from build123d import *

# Parameters (mm, degrees)
BOSS_EXTRUDE1_DEPTH = 15
SHELL2_T            = 6
CUT_EXTRUDE1_REACH  = 17
SKETCH2_R           = 15
CUT_EXTRUDE2_REACH  = 42
SKETCH3_R           = 2.25
SKETCH5_R           = 5.54
CUT_EXTRUDE3_DEPTH  = 21


with BuildPart() as part:
    # Sketch1 → Boss-Extrude1 (new body)
    with BuildSketch(Plane.XY):
        with BuildLine():
            Line((-25, 0), (-25, -15))
            Line((-25, -15), (25, -15))
            Line((25, -15), (25, 0))
            ThreePointArc((25, 0), (0, 25), (-25, 0))
        make_face()
    extrude(amount=BOSS_EXTRUDE1_DEPTH)

    # Shell2 (no face opened: a closed hollow body)
    add(offset(amount=-SHELL2_T, mode=Mode.PRIVATE), mode=Mode.SUBTRACT)

    # Sketch2 → Cut-Extrude1 (cut, up to next)
    with BuildSketch(Plane.XY.offset(15), mode=Mode.PRIVATE) as cut_extrude1_sk1:
        with Locations((0, -5)):
            Circle(SKETCH2_R)
    cut_extrude1_tool1 = extrude(cut_extrude1_sk1.sketch, amount=-CUT_EXTRUDE1_REACH, mode=Mode.PRIVATE) & part.part
    add(cut_extrude1_tool1.solids().sort_by_distance((0, -5, 15))[0], mode=Mode.SUBTRACT)

    # Sketch3 → Cut-Extrude2 (cut, up to next)
    with BuildSketch(Plane(origin=(0, 25, 0), x_dir=(1, 0, 0), z_dir=(0, 1, 0)), mode=Mode.PRIVATE) as cut_extrude2_sk1:
        with Locations((-19, -7.5)):
            Circle(SKETCH3_R)
    cut_extrude2_tool1 = extrude(cut_extrude2_sk1.sketch, amount=-CUT_EXTRUDE2_REACH, mode=Mode.PRIVATE) & part.part
    add(cut_extrude2_tool1.solids().sort_by_distance((-19, 25, 7.5))[0], mode=Mode.SUBTRACT)
    # Sketch3 → Cut-Extrude2 (cut, up to next)
    with BuildSketch(Plane(origin=(0, 25, 0), x_dir=(1, 0, 0), z_dir=(0, 1, 0)), mode=Mode.PRIVATE) as cut_extrude2_sk2:
        with Locations((19, -7.5)):
            Circle(SKETCH3_R)
    cut_extrude2_tool2 = extrude(cut_extrude2_sk2.sketch, amount=-CUT_EXTRUDE2_REACH, mode=Mode.PRIVATE) & part.part
    add(cut_extrude2_tool2.solids().sort_by_distance((19, 25, 7.5))[0], mode=Mode.SUBTRACT)

    # Sketch5 → Cut-Extrude3 (cut)
    with BuildSketch(Plane(origin=(0, 25, 0), x_dir=(1, 0, 0), z_dir=(0, 1, 0))):
        with Locations((19, -7.5)):
            Circle(SKETCH5_R)
        with Locations((-19, -7.5)):
            Circle(SKETCH5_R)
    extrude(amount=-CUT_EXTRUDE3_DEPTH, mode=Mode.SUBTRACT)


solid = part.part
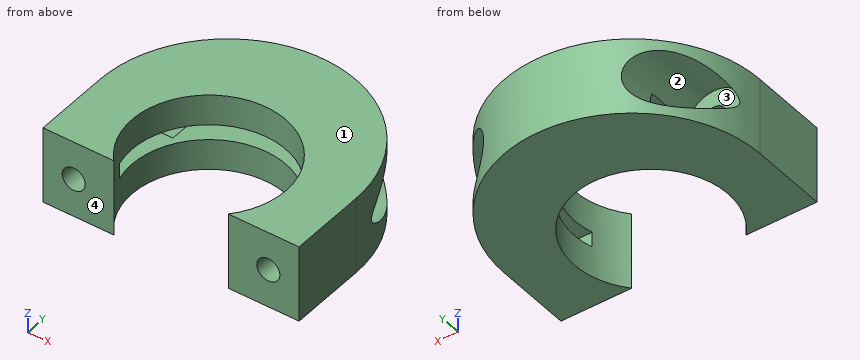
Here's how the part is built. I have some questions about the finished solid (model axes, mm). Face numbers are marked on the shaded views. Round coordinates to 2 decimals unless told otherwise and drop trailing zeros. Loops run counter-clockwise (first coordinate to the right, second up) from the corner with the lowest first, then second, coordinate; pieces in that order, holes last. Notation, with made-up numbers: M 41,-23 L 88,-23 A22 cw 88,1 Z; hole C 46,86.25 d6. An arc over 180 degrees is marked long. Write each question's results on one line, items separated by ' | '. Start each with the question number.
(1) I want a section at C-C (z = 7.5). Please give me the cut outline in (x, y), then the cut area to 3 significant figures.
(2) I want a section at D-D (x = -19). Please give me the cut outline in (y, z).
(3) I want a section at B-B (x = 0). Please give me the cut outline in (y, z).
(4) Thinking about a two-plate mould opening in Z: for the marked faces 1, 2, 3 and 4, which applies, pulls with the +Z half, pulls with the -Z half, needs draft (parallel to the pull), parting line crosses it, or undercut?
(5) I want a section at A-A (y = -5). Please give me the cut outline in (x, z), then the cut area to 3 significant figures.
(6) If I drill on probe 1 along X at (y, z) = (-5.5, 7.5); probe 2 along X at (y, z) = (3.5, 5.5); probe 3 along Z at (x, y) = (-19, -6.5), over which ranges is the centre line in solid material (lowest first)? Write a range as from..to.
(7) Will these pins go through, and if not, where does the flat tip stop? P1, Ø0.9, axis at x = -15.5, z = 8, coming from the +Y side; P2, Ø1, axis at y = 21, z = 5, coming from the +X side; P3, Ø5.5, axis at x = 18, z = 5.5, coming from the +Y side; P4, Ø24, axis at x = 0, y = -5, coming from the -Z side.
Solved:
1) outline: M -25,-15 L -21.25,-15 L -21.25,4 L -24.54,4 L -24.54,4.77 A25 ccw -25,0 Z; M -16.75,-15 L -11.18,-15 A15 cw -14.46,-9 L -16.75,-9 Z; M -13.46,13.41 A19 cw 13.46,13.41 L 13.46,21.07 A25 ccw -13.46,21.07 Z; M 11.18,-15 L 16.75,-15 L 16.75,-9 L 14.46,-9 A15 cw Z; M 21.25,-15 L 25,-15 L 25,0 A25 ccw 24.54,4.77 L 24.54,4 L 21.25,4 Z | area: 360 mm²
2) outline: M -15,0 L 16.25,0 L 16.25,1.96 L 4,1.96 L 4,5.25 L -15,5.25 Z; M -15,9.75 L 4,9.75 L 4,13.04 L 16.25,13.04 L 16.25,15 L -15,15 Z
3) outline: M 10,0 L 25,0 L 25,15 L 10,15 L 10,9 L 19,9 L 19,6 L 10,6 Z
4) face 1: pulls with the +Z half | face 2: undercut | face 3: undercut | face 4: needs draft
5) outline: M -25,0 L -15,0 L -15,6 L -17.32,6 A2.25 cw long -17.32,9 L -15,9 L -15,15 L -25,15 Z; M 15,0 L 25,0 L 25,15 L 15,15 L 15,9 L 17.32,9 A2.25 cw long 17.32,6 L 15,6 Z | area: 257 mm²
6) probe 1: x = -25..-21.25, 21.25..25 | probe 2: x = -24.75..-20.03, -17.97..-12.36, 12.36..17.97, 20.03..24.75 | probe 3: z = 0..5.25, 9.75..15
7) P1: stops at y = -9 | P2: stops at x = 14.2 | P3: stops at y = 4 | P4: passes through
